from build123d import *

# Parameters (mm, degrees)
F0_R      = 0.016454
F1_DEPTH  = 0.127
F0_R_2    = 0.030793
F2_DEPTH  = 0.254
F0_R_3    = 0.044201
F3_DEPTH  = 0.381
F0_R_4    = 0.058333
F4_DEPTH  = 0.508
F0_R_5    = 0.082289
F5_DEPTH  = 0.635
F0_R_6    = 0.110964
F6_DEPTH  = 0.762
F0_R_7    = 0.166573
F7_DEPTH  = 1.016
F0_R_8    = 0.219095
F8_DEPTH  = 1.27
F0_R_9    = 0.274683
F9_DEPTH  = 1.524
F0_R_10   = 0.337165
F10_DEPTH = 1.651
F0_R_11   = 0.408015
F11_DEPTH = 1.778
F0_R_12   = 0.485557
F12_DEPTH = 1.905
F0_R_13   = 0.578509
F13_DEPTH = 2.032
F0_R_14   = 0.667796
F14_DEPTH = 2.159
F0_R_15   = 0.802034
F15_DEPTH = 2.286
F0_R_16   = 1.032953
F16_DEPTH = 2.413
F0_R_17   = 1.576552
F17_DEPTH = 2.54
F0_R_18   = 2.397447
F18_DEPTH = 3.81
F0_R_19   = 3.303479
F19_DEPTH = 4.445
F0_R_20   = 4.231249
F20_DEPTH = 5.08
F0_R_21   = 5.202771
F21_DEPTH = 6.35
F0_R_22   = 6.121839
F22_DEPTH = 6.985
F0_R_23   = 7.050554
F23_DEPTH = 7.62
F0_R_24   = 7.944104
F24_DEPTH = 7.62
F0_R_25   = 8.922677
F25_DEPTH = 8.89
F0_R_26   = 9.808018
F26_DEPTH = 10.16
F0_R_27   = 10.844167
F27_DEPTH = 12.7
F0_R_28   = 11.761567
F28_DEPTH = 15.24
F0_R_29   = 12.626264
F29_DEPTH = 17.78
F0_R_30   = 13.574891
F30_DEPTH = 20.32
F0_R_31   = 14.58843
F31_DEPTH = 22.86
F0_R_32   = 15.648071
F32_DEPTH = 25.4
F0_R_33   = 16.614679
F33_DEPTH = 27.94
F0_R_34   = 17.602132
F34_DEPTH = 30.48
F0_R_35   = 18.606067
F35_DEPTH = 33.02
F0_R_36   = 19.616036
F36_DEPTH = 35.56
F0_R_37   = 20.71569
F37_DEPTH = 38.1
F0_R_38   = 21.775007
F38_DEPTH = 40.64
F0_R_39   = 22.809828
F39_DEPTH = 43.18


with BuildPart() as f1:
    # F0 (on Top) → F1 (new body)
    with BuildSketch(Plane.XY):
        Circle(F0_R)
    extrude(amount=F1_DEPTH)

    # F0 (on Top) → F2 (join)
    with BuildSketch(Plane.XY):
        Circle(F0_R_2)
        Circle(F0_R, mode=Mode.SUBTRACT)
    extrude(amount=F2_DEPTH)

    # F0 (on Top) → F3 (join)
    with BuildSketch(Plane.XY):
        Circle(F0_R_3)
        Circle(F0_R_2, mode=Mode.SUBTRACT)
    extrude(amount=F3_DEPTH)

    # F0 (on Top) → F4 (join)
    with BuildSketch(Plane.XY):
        Circle(F0_R_4)
        Circle(F0_R_3, mode=Mode.SUBTRACT)
    extrude(amount=F4_DEPTH)

    # F0 (on Top) → F5 (join)
    with BuildSketch(Plane.XY):
        Circle(F0_R_5)
        Circle(F0_R_4, mode=Mode.SUBTRACT)
    extrude(amount=F5_DEPTH)

    # F0 (on Top) → F6 (join)
    with BuildSketch(Plane.XY):
        Circle(F0_R_6)
        Circle(F0_R_5, mode=Mode.SUBTRACT)
    extrude(amount=F6_DEPTH)

    # F0 (on Top) → F7 (join)
    with BuildSketch(Plane.XY):
        Circle(F0_R_7)
        Circle(F0_R_6, mode=Mode.SUBTRACT)
    extrude(amount=F7_DEPTH)

    # F0 (on Top) → F8 (join)
    with BuildSketch(Plane.XY):
        Circle(F0_R_8)
        Circle(F0_R_7, mode=Mode.SUBTRACT)
    extrude(amount=F8_DEPTH)

    # F0 (on Top) → F9 (join)
    with BuildSketch(Plane.XY):
        Circle(F0_R_9)
        Circle(F0_R_8, mode=Mode.SUBTRACT)
    extrude(amount=F9_DEPTH)

    # F0 (on Top) → F10 (join)
    with BuildSketch(Plane.XY):
        Circle(F0_R_10)
        Circle(F0_R_9, mode=Mode.SUBTRACT)
    extrude(amount=F10_DEPTH)

    # F0 (on Top) → F11 (join)
    with BuildSketch(Plane.XY):
        Circle(F0_R_11)
        Circle(F0_R_10, mode=Mode.SUBTRACT)
    extrude(amount=F11_DEPTH)

    # F0 (on Top) → F12 (join)
    with BuildSketch(Plane.XY):
        Circle(F0_R_12)
        Circle(F0_R_11, mode=Mode.SUBTRACT)
    extrude(amount=F12_DEPTH)

    # F0 (on Top) → F13 (join)
    with BuildSketch(Plane.XY):
        Circle(F0_R_13)
        Circle(F0_R_12, mode=Mode.SUBTRACT)
    extrude(amount=F13_DEPTH)

    # F0 (on Top) → F14 (join)
    with BuildSketch(Plane.XY):
        Circle(F0_R_14)
        Circle(F0_R_13, mode=Mode.SUBTRACT)
    extrude(amount=F14_DEPTH)

    # F0 (on Top) → F15 (join)
    with BuildSketch(Plane.XY):
        Circle(F0_R_15)
        Circle(F0_R_14, mode=Mode.SUBTRACT)
    extrude(amount=F15_DEPTH)

    # F0 (on Top) → F16 (join)
    with BuildSketch(Plane.XY):
        Circle(F0_R_16)
        Circle(F0_R_15, mode=Mode.SUBTRACT)
    extrude(amount=F16_DEPTH)

    # F0 (on Top) → F17 (join)
    with BuildSketch(Plane.XY):
        Circle(F0_R_17)
        Circle(F0_R_16, mode=Mode.SUBTRACT)
    extrude(amount=F17_DEPTH)

    # F0 (on Top) → F18 (join)
    with BuildSketch(Plane.XY):
        Circle(F0_R_18)
        Circle(F0_R_17, mode=Mode.SUBTRACT)
    extrude(amount=F18_DEPTH)

    # F0 (on Top) → F19 (join)
    with BuildSketch(Plane.XY):
        Circle(F0_R_19)
        Circle(F0_R_18, mode=Mode.SUBTRACT)
    extrude(amount=F19_DEPTH)

    # F0 (on Top) → F20 (join)
    with BuildSketch(Plane.XY):
        Circle(F0_R_20)
        Circle(F0_R_19, mode=Mode.SUBTRACT)
    extrude(amount=F20_DEPTH)

    # F0 (on Top) → F21 (join)
    with BuildSketch(Plane.XY):
        Circle(F0_R_21)
        Circle(F0_R_20, mode=Mode.SUBTRACT)
    extrude(amount=F21_DEPTH)

    # F0 (on Top) → F22 (join)
    with BuildSketch(Plane.XY):
        Circle(F0_R_22)
        Circle(F0_R_21, mode=Mode.SUBTRACT)
    extrude(amount=F22_DEPTH)

    # F0 (on Top) → F23 (join)
    with BuildSketch(Plane.XY):
        Circle(F0_R_23)
        Circle(F0_R_22, mode=Mode.SUBTRACT)
    extrude(amount=F23_DEPTH)

    # F0 (on Top) → F24 (join)
    with BuildSketch(Plane.XY):
        Circle(F0_R_24)
        Circle(F0_R_23, mode=Mode.SUBTRACT)
    extrude(amount=F24_DEPTH)

    # F0 (on Top) → F25 (join)
    with BuildSketch(Plane.XY):
        Circle(F0_R_25)
        Circle(F0_R_24, mode=Mode.SUBTRACT)
    extrude(amount=F25_DEPTH)

    # F0 (on Top) → F26 (join)
    with BuildSketch(Plane.XY):
        Circle(F0_R_26)
        Circle(F0_R_25, mode=Mode.SUBTRACT)
    extrude(amount=F26_DEPTH)

    # F0 (on Top) → F27 (join)
    with BuildSketch(Plane.XY):
        Circle(F0_R_27)
        Circle(F0_R_26, mode=Mode.SUBTRACT)
    extrude(amount=F27_DEPTH)

    # F0 (on Top) → F28 (join)
    with BuildSketch(Plane.XY):
        Circle(F0_R_28)
        Circle(F0_R_27, mode=Mode.SUBTRACT)
    extrude(amount=F28_DEPTH)

    # F0 (on Top) → F29 (join)
    with BuildSketch(Plane.XY):
        Circle(F0_R_29)
        Circle(F0_R_28, mode=Mode.SUBTRACT)
    extrude(amount=F29_DEPTH)

    # F0 (on Top) → F30 (join)
    with BuildSketch(Plane.XY):
        Circle(F0_R_30)
        Circle(F0_R_29, mode=Mode.SUBTRACT)
    extrude(amount=F30_DEPTH)

    # F0 (on Top) → F31 (join)
    with BuildSketch(Plane.XY):
        Circle(F0_R_31)
        Circle(F0_R_30, mode=Mode.SUBTRACT)
    extrude(amount=F31_DEPTH)

    # F0 (on Top) → F32 (join)
    with BuildSketch(Plane.XY):
        Circle(F0_R_32)
        Circle(F0_R_31, mode=Mode.SUBTRACT)
    extrude(amount=F32_DEPTH)

    # F0 (on Top) → F33 (join)
    with BuildSketch(Plane.XY):
        Circle(F0_R_33)
        Circle(F0_R_32, mode=Mode.SUBTRACT)
    extrude(amount=F33_DEPTH)

    # F0 (on Top) → F34 (join)
    with BuildSketch(Plane.XY):
        Circle(F0_R_34)
        Circle(F0_R_33, mode=Mode.SUBTRACT)
    extrude(amount=F34_DEPTH)

    # F0 (on Top) → F35 (join)
    with BuildSketch(Plane.XY):
        Circle(F0_R_35)
        Circle(F0_R_34, mode=Mode.SUBTRACT)
    extrude(amount=F35_DEPTH)

    # F0 (on Top) → F36 (join)
    with BuildSketch(Plane.XY):
        Circle(F0_R_36)
        Circle(F0_R_35, mode=Mode.SUBTRACT)
    extrude(amount=F36_DEPTH)

    # F0 (on Top) → F37 (join)
    with BuildSketch(Plane.XY):
        Circle(F0_R_37)
        Circle(F0_R_36, mode=Mode.SUBTRACT)
    extrude(amount=F37_DEPTH)

    # F0 (on Top) → F38 (join)
    with BuildSketch(Plane.XY):
        Circle(F0_R_38)
        Circle(F0_R_37, mode=Mode.SUBTRACT)
    extrude(amount=F38_DEPTH)

    # F0 (on Top) → F39 (join)
    with BuildSketch(Plane.XY):
        Circle(F0_R_39)
        Circle(F0_R_38, mode=Mode.SUBTRACT)
    extrude(amount=F39_DEPTH)


solid = f1.part
Geometry check sheet. Reference: the model listing, model coordinates, mm. A direction names the side the tool comes from. Give positions to 0.01 mm unless a question says otherwise; leave off trailing zeros. Loops run counter-clockwise (first coordinate to the right, second up) from the corner with the lowest first, then second, coordinate; pieces in that order, holes last. Notation, with made-up numbers: (-31, -5.75) -> (-11, -5.75) arc R20 ccw to (-11, 10.25) -> close; hole circle Ø3 at (-6, -33). An arc over 180 degrees is marked (long way). Answer in a Markdown table with one row per item. Add a question column.
1) Gauge pin test, flat ends, axial feed: P1, Ø12, axis at y = -7, z = 28.5, coming from the -X side; P2, Ø4, axis at x = -13, z = 25.5, coming from the -Y side; P3, Ø3, axis at x = 0, y = 0, coming from the +Z side. Record the tip position at first contact, or that the pin passes through.
2) Cross-section at B-B on z = 27. Record the boundary of the cut face in (x, y), and give its area (3 significant figures).
3) Material ranges on probe 1 along Y at (x, z) = (0, 10.5); probe 2 along Y at (x, z) = (0, 33.65); probe 3 along Z at (x, y) = (18.5, -0.5), recorded low to high. Write a range as from..to.
4) Set-up check for faces 1 (the face through (-14.765, -11.322, 34.272)), 2 (the face through (0, -22, 43.18)): record each of +Z, -Z, +X, -X, +Y, -Y from which the full face is reachable in a straight line by a thin tool's end or side.
5) Cross-section at A-A on z = 18.5. Record the boundary of the cut face in (x, y), and give its area (3 significant figures).
6) Draft check along Y on faces 3 (the face through (-0.3, 0.3, 0)), 4 (the face through (-2.969, 22.616, 21.288)), 5 (the face through (-3, -5, 6.985)). Enter one of: pulls with the +Y half, pulls with the -Y half, needs draft (parallel to the pull), parting line crosses it, or undercut.
Outcome:
| question | item | result |
|---|---|---|
| 1 | P1 | stops at x = -22.79 |
| 1 | P2 | stops at y = -19.98 |
| 1 | P3 | stops at z = 2.54 |
| 2 | outline | circle Ø45.62 at (0, 0); hole circle Ø31.3 at (0, 0) |
| 2 | area | 865 mm^2 |
| 3 | probe 1 | y = -22.81..-9.81, 9.81..22.81 |
| 3 | probe 2 | y = -22.81..-18.61, 18.61..22.81 |
| 3 | probe 3 | z = 0..33.02 |
| 4 | face 1 | +Z |
| 4 | face 2 | +Z, +X, -X, +Y, -Y |
| 5 | outline | circle Ø45.62 at (0, 0); hole circle Ø25.25 at (0, 0) |
| 5 | area | 1,130 mm^2 |
| 6 | face 3 | needs draft |
| 6 | face 4 | parting line crosses it |
| 6 | face 5 | undercut |
